Study the drawing (mm; zero at the part's minimum x, y, z) and answer. A direction names the side the tool comes from. Give positions to 0.01 mm unless a question says otherwise; leave off trailing zeros. Order: outer loops, then holes, each group sorted by start corner. A loop starts at its lowest first (then second) coordinate and runs counter-clockwise, first axis right, second up.
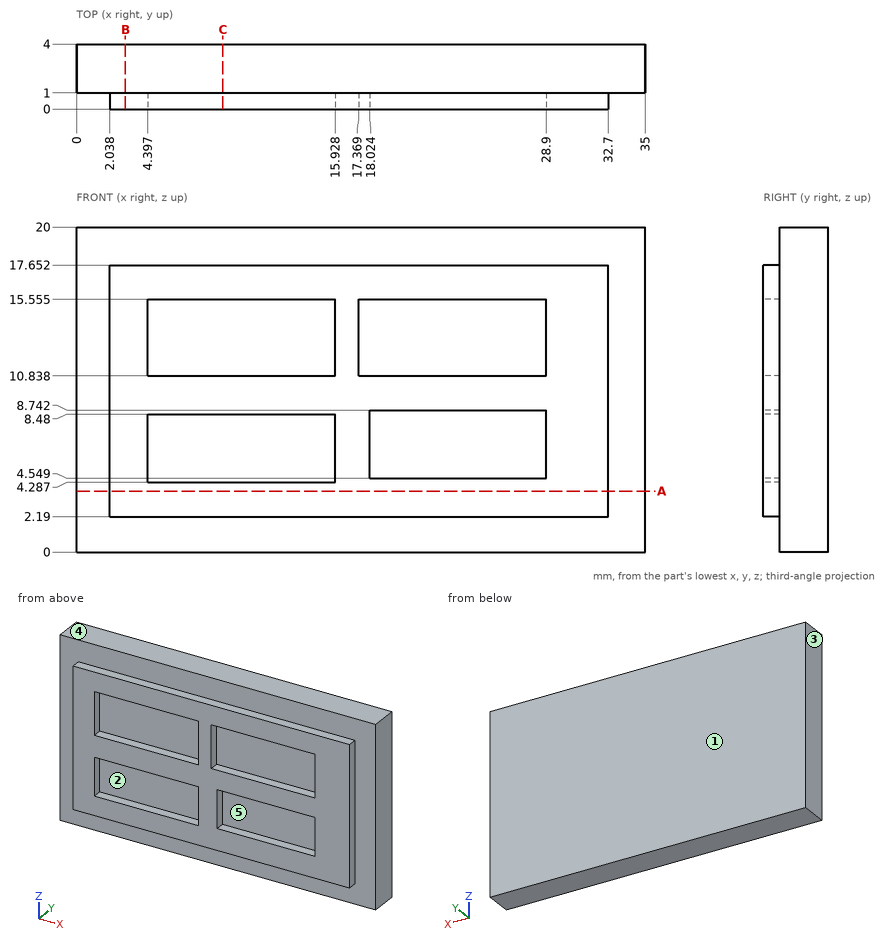
1) For a pull along X with two mould halves and no side action, classify the marked faces 3, 4 and 5 as +X half, -X half, draft (parallel to the pull), parting line (faces both ways), or undercut.
Geometry says:
face 3: -X half
face 4: draft
face 5: undercut
2) Find section C-C (x = 9). Write down the section's boundary in (y, z) (1 decimal).
Geometry says:
outline: (0, 2.2) - (1, 2.2) - (1, 0) - (4, 0) - (4, 20) - (1, 20) - (1, 17.7) - (0, 17.7) - (0, 15.6) - (1, 15.6) - (1, 10.8) - (0, 10.8) - (0, 8.5) - (1, 8.5) - (1, 4.3) - (0, 4.3) - close
3) Find section A-A (z = 3.75). Write down the section's boundary in (x, y), then the cut area to 3 significant figures.
Geometry says:
outline: (0, 1) - (2.04, 1) - (2.04, 0) - (32.7, 0) - (32.7, 1) - (35, 1) - (35, 4) - (0, 4) - close
area: 136 mm2
4) A tool of negligible diameter and unlimited length cuts with its end or side. For the marked faces 1 and 2, from which of +Z, -Z, +X, -X, +Y, -Y can it reach the whole face along a straight path? Write none if from no direction.
Geometry says:
face 1: +Z, -Z, +X, -X, +Y
face 2: -Y
5) Straight lines are drawn through the part: probe 1 along Z at (x, y) = (13.5, 0.2) (1 decimal); probe 2 along Y at (x, z) = (15, 17.75); probe 3 along X at (y, z) = (0.25, 9.5). For each, find the intervals that lie inside material, in ascending order.
Geometry says:
probe 1: z = 2.2 to 4.3, 8.5 to 10.8, 15.6 to 17.7
probe 2: y = 1 to 4
probe 3: x = 2.04 to 32.7
6) Given P1, Ø0.8, axis at x = 16, y = 0.5, coming from the +Z side; P2, Ø2.5, axis at x = 10.5, z = 13, coming from the -Y side; P3, Ø0.8, axis at x = 12.5, y = 0.5, coming from the -Z side, each flat-ended and moving along its own axis, determine where each tip first touches the part or whether it passes through.
Geometry says:
P1: stops at z = 17.65
P2: stops at y = 1
P3: stops at z = 2.19
7) Find section B-B (x = 3). Write down the section's boundary in (y, z).
Geometry says:
outline: (0, 2.19) - (1, 2.19) - (1, 0) - (4, 0) - (4, 20) - (1, 20) - (1, 17.65) - (0, 17.65) - close
